```python
from build123d import *

# Parameters (mm, degrees)
VACIADO1_T              = -0.5
CROQUIS3_W              = 20
CROQUIS3_H              = 15
SALIENTE_EXTRUIR1_DEPTH = 3


with BuildPart() as part:
    # Croquis1 → Revolución1 (revolve)
    with BuildSketch(Plane.XY):
        with BuildLine():
            Line((5.855337127, 0), (-5.144662873, 0))
            Line((-5.144662873, 0), (-5.144662873, 5.744562647))
            ThreePointArc((-5.144662873, 5.744562647), (2.095707476, 6.204836823), (5.855337127, 0))
        make_face()
    revolve(axis=Axis((5.855337127, 0, 0), (-1, 0, 0)))

    # Vaciado1
    vaciado1_openings = [part.faces().sort_by_distance(p)[0] for p in [
        (-5.144662873, 0, 0),
    ]]
    offset(amount=VACIADO1_T, openings=vaciado1_openings, kind=Kind.INTERSECTION)

    # Croquis2 → Revolución2 (revolve)
    with BuildSketch(Plane.XY, mode=Mode.PRIVATE) as revoluci_n2_sk:
        with BuildLine():
            Line((5.855337127, 0), (9.355337127, 0))
            Line((9.355337127, 0), (9.355337127, -7.5))
            Line((9.355337127, -7.5), (7.115337127, -7.5))
            ThreePointArc((7.115337127, -7.5), (6.711500505, -4.686879238), (5.532607443, -2.100966713))
            Line((5.532607443, -2.100966713), (5.855337127, 0))
        make_face()
    revolve(revoluci_n2_sk.sketch.rotate(Axis((0, 0, 0), (1, 0, 0)), 180), axis=Axis((0, 0, 0), (1, 0, 0)))

    # Croquis3 → Saliente-Extruir1 (add)
    with BuildSketch(Plane(origin=(9.355337127, 0, 0), x_dir=(0, 0, -1), z_dir=(1, 0, 0))):
        Rectangle(CROQUIS3_W, CROQUIS3_H)
    extrude(amount=SALIENTE_EXTRUIR1_DEPTH)


solid = part.part
```
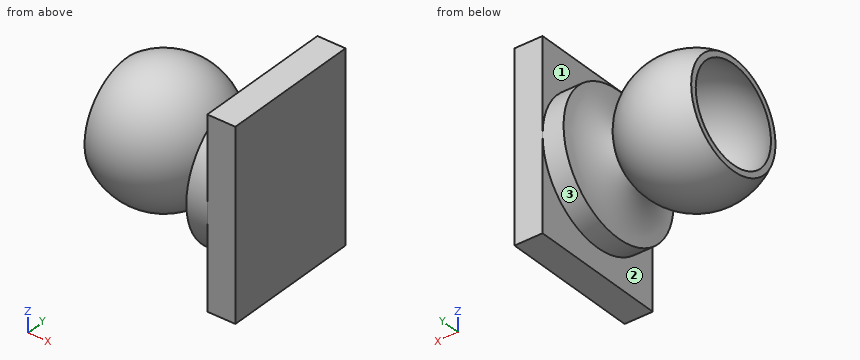
Geometry check sheet. Reference: the model listing, model coordinates, mm. Face numbers are marked on the shaded views. A direction names the side the tool comes from. Coordinates: 2 decimals unless noted, no trailing zeros. Order: outer loops, then holes, each group sorted by start corner. A loop starts at its lowest first (then second) coordinate and runs counter-clockwise, first axis right, second up. Notation, with made-up numbers: (-32.5, 80.25) - (2.5, 80.25) arc R18 cw to (2.5, 94.25) - close; hole circle Ø7 at (-15, 29.25). An arc over 180 degrees is marked (long way). Answer as a JSON object with one key per item and string values. Group by question number.
Item 1: Sectioned sample at B-B, the plane z = -8.5. Record the cut outline in (x, y).
Item 2: Depth check by flat-ended pin: pin 1 Ø1 at (x, y) = (0, -3) entering from +Z; pin 2 Ø8 at (x, y) = (5, 5) entering from +Z; pin 3 Ø1 at (y, z) = (1.5, -4) entering from -X. Enter the tip coordinate at first touch or a pass-through.
Item 3: Sectioned sample at A-A, the plane x = 9. Record the cut outline in (y, z), and give its area (3 significant figures).
Item 4: Tool access check on the marked faces 1, 2 and 3. Record the directions out of +Z, -Z, +X, -X, +Y, -Y that give a thin tool (end or side, any length) a straight path to the whole face; none if there is none.
Item 5: Sectioned sample at C-C, the plane x = 5. Record the cut outline in (y, z).
Item 6: Scan lines: probe 1 along X at (y, z) = (0.5, -5.5); probe 2 along X at (y, z) = (-2, 5.5); probe 3 along X at (y, z) = (6.75, -4.5). Record each from-to range of solid material in increasing order.
Resolved:
{
 "1": {"outline": "(9.36, -7.5) - (12.36, -7.5) - (12.36, 7.5) - (9.36, 7.5) - close"},
 "2": {"pin 1": "z = 6.45", "pin 2": "z = 7.33", "pin 3": "x = 3.27"},
 "3": {"outline": "circle Ø15 at (0, 0)", "area": "177 mm^2"},
 "4": {"face 1": "+Z, -X", "face 2": "-Z, -X", "face 3": "-X"},
 "5": {"outline": "circle Ø6.71 at (0, 0); hole circle Ø4.24 at (0, 0)"},
 "6": {"probe 1": "-5.14 to -4.57, 2.28 to 3.16, 6.92 to 12.36", "probe 2": "-4.99 to -3.97, 1.68 to 2.7, 6.98 to 12.36", "probe 3": "9.36 to 12.36"}
}
